Part model, mm, in its own coordinate system. Face numbers are marked on the shaded views. A direction names the side the tool comes from. Give positions to 0.01 mm unless a question says otherwise; leave off trailing zeros. Order: outer loops, then holes, each group sorted by start corner. A loop starts at its lowest first (then second) coordinate and runs counter-clockwise, first axis right, second up. Notation, with made-up numbers: (-35.75, 79) - (17.25, 79) arc R18 ccw to (17.25, 114) - close; hole circle Ø5 at (-39, 62). An arc over 180 degrees is marked (long way). One line per item, written item: value.
```python
from build123d import *

# Parameters (mm, degrees)
SKETCH1_W           = 100
SKETCH1_H           = 150
BOSS_EXTRUDE1_DEPTH = 80
SKETCH2_OUTSIDE_W   = 141.446
SKETCH2_OUTSIDE_H   = 121.446
CUT_EXTRUDE2_DEPTH  = 50
SKETCH4_OUTSIDE_W   = 191.446
SKETCH4_OUTSIDE_H   = 121.446
CUT_EXTRUDE3_DEPTH  = 100


with BuildPart() as part:
    # Sketch1 → Boss-Extrude1 (new body)
    with BuildSketch(Plane(origin=(0, 0, 0), x_dir=(1, 0, 0), z_dir=(0, 1, 0))):
        Rectangle(SKETCH1_W, SKETCH1_H)
    extrude(amount=BOSS_EXTRUDE1_DEPTH)

    # Sketch2 outside → Cut-Extrude2 (cut)
    with BuildSketch(Plane.XY.offset(75)):
        with Locations((0, 40)):
            Rectangle(SKETCH2_OUTSIDE_W, SKETCH2_OUTSIDE_H)
        Polygon((50, 0), (-50, 0), (-50, 80), (-25, 80), (0, 35), (25, 80), (50, 80), align=None, mode=Mode.SUBTRACT)
    extrude(amount=-CUT_EXTRUDE2_DEPTH, mode=Mode.SUBTRACT)

    # Sketch4 outside → Cut-Extrude3 (cut)
    with BuildSketch(Plane.ZY.offset(50)):
        with Locations((0, 40)):
            Rectangle(SKETCH4_OUTSIDE_W, SKETCH4_OUTSIDE_H)
        Polygon((-75, 80), (-50, 80), (-50, 60), (-30, 60), (-30, 40), (-10, 40), (-10, 60), (15, 60), (15, 80), (75, 80), (75, 0), (-75, 0), align=None, mode=Mode.SUBTRACT)
    extrude(amount=-CUT_EXTRUDE3_DEPTH, mode=Mode.SUBTRACT)


solid = part.part
```
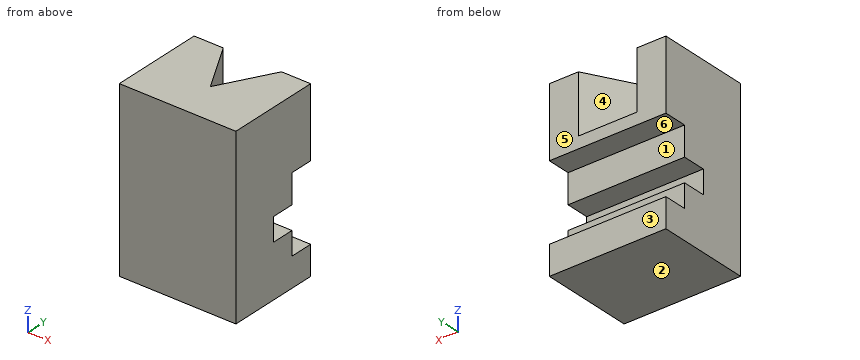
1) Slice it at D-D on x = 19. Write the cut outline in (y, z).
Answer:
outline: (0, -75) - (80, -75) - (80, -50) - (60, -50) - (60, -30) - (40, -30) - (40, -10) - (60, -10) - (60, 15) - (80, 15) - (80, 25) - (69.2, 25) - (69.2, 75) - (0, 75) - close
2) Drop flat-ended pins along their axis: P1, Ø4, axis at x = 37, z = -13.5, coming from the +Y side; P2, Ø22, axis at x = -13, z = -20.5, coming from the +Y side. Give the stop position or say it passes through.
Answer:
P1: stops at y = 40
P2: stops at y = 60
3) Wall check: line 1 along Z through (x, y) = (25, 68); line 2 along Z through (x, y) = (-13.5, 63); line 3 along Y through (x, z) = (-1.5, -23). Give the ranges that are in metal, low to high. Write a range as [from, to].
Answer:
line 1: z = [-75, -50], [15, 75]
line 2: z = [-75, -50], [15, 25]
line 3: y = [0, 40]
4) Slice it at A-A on x = 9. Write the cut outline in (y, z), then the cut area to 3 significant figures.
Answer:
outline: (0, -75) - (80, -75) - (80, -50) - (60, -50) - (60, -30) - (40, -30) - (40, -10) - (60, -10) - (60, 15) - (80, 15) - (80, 25) - (51.2, 25) - (51.2, 75) - (0, 75) - close
area: 8,860 mm2
5) Slice it at B-B on z = 50. Write the cut outline in (x, y).
Answer:
outline: (-50, 0) - (50, 0) - (50, 80) - (25, 80) - (0, 35) - (-25, 80) - (-50, 80) - close
6) Slice it at C-C on y = 51. Write the cut outline in (x, z).
Answer:
outline: (-50, -75) - (50, -75) - (50, -30) - (-50, -30) - close; (-50, -10) - (50, -10) - (50, 75) - (8.89, 75) - (8.89, 25) - (-8.89, 25) - (-8.89, 75) - (-50, 75) - close
7) Which spindle directions (+Z, -Z, +X, -X, +Y, -Y) get a long thin tool onto all of the face, cutting with end or side? Do the marked faces 4, 5 and 6. Say none if no direction does.
Answer:
face 4: +Z, +Y
face 5: +Z, -Z, +X, -X, +Y
face 6: +X, -X, +Y
8) Two-plate mould, pull along Z, no slides. Class the marked faces 1, 2 and 3: pulls with the +Z half, pulls with the -Z half, needs draft (parallel to the pull), parting line crosses it, or undercut.
Answer:
face 1: undercut
face 2: pulls with the -Z half
face 3: needs draft
